Autodesk Inventor part; units mm, degrees
ref_plane "YZ Plane" through (0, 0, 0) normal (1, 0, 0) x (0, 1, 0)
ref_plane "XZ Plane" through (0, 0, 0) normal (0, 1, 0) x (-1, 0, 0)
ref_plane "XY Plane" through (0, 0, 0) normal (0, 0, 1) x (1, 0, 0)
sketch "Sketch1" plane through (0, 0, 0) normal (0, 1, 0) x (-1, 0, 0)
  line L0 (-9.1057, 3.648) -> (-9.1057, -9.552)
  line L1 (4.8943, -9.552) -> (4.8943, 8.308)
  line L2 (4.8943, 8.308) -> (-9.1057, 3.648)
  line L3 (-2.1057, 5.978) -> (-2.1057, 1.978)
  circle A0 centre (-2.1057, 0.378) radius 1.6
  line L4 (4.8943, -9.552) -> (4.8943, -12.052)
  line L5 (-9.1057, -9.552) -> (-9.1057, -12.052)
  line L6 (4.8943, -12.052) -> (-9.1057, -12.052)
  circle A1 centre (-2.1057, -12.052) radius 4
  line L7 (-2.1057, -1.222) -> (-2.1057, -8.052)
  line L8 (4.8943, 1.978) -> (-2.1057, 1.978)
  line L9 (-9.1057, 1.978) -> (-2.1057, 1.978)
  point P0 (0, 0)
  point P1 (1.8943, -12.052)
  point P2 (-6.1057, -12.052)
  dimension "d8" = 3.2
  dimension "d19" = 8
  dimension "d5" = 13.2
  dimension "d6" = 4
  dimension "d10" = 17.86
  dimension "d13" = 14
  dimension "d16" = 2.5
extrude "Extrusion2" add sketch "Sketch1" along normal blind 4 contours L2 L3 L9 L0 | L9 A0 L7 A1 L6 L5 L0 | L2 L1 L8 L3 | L8 L1 L4 L6 A1 L7 A0
sketch "Sketch2" plane through (0, 0, 0) normal (0, -1, 0) x (1, 0, 0)
  line L0 (9.1057, 3.648) -> (9.1057, -12.052)
  line L1 (9.1057, 2.0387) -> (-4.8943, 2.0387)
  line L2 (-4.8943, -12.052) -> (-4.8943, 8.308)
  line L3 (-4.8943, 2.0387) -> (-4.8943, 8.308)
  line L4 (-4.8943, 8.308) -> (9.1057, 3.648)
  line L5 (-4.8943, 8.308) -> (9.1057, 3.648)
  line L6 (9.1057, 3.648) -> (9.1057, 2.0387)
  point P0 (0, 0)
extrude "Extrusion3" add sketch "Sketch2" against normal blind 6
properties part number "plungerholdermod2"
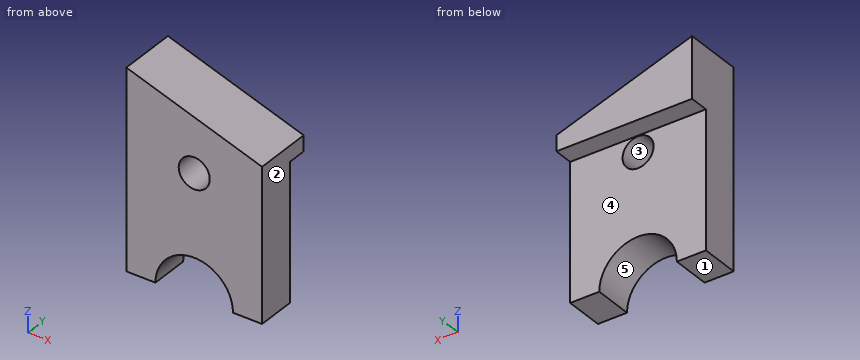
CAD build for the part. Positions are in the model's coordinates, mm. Face numbers are marked on the shaded views. A direction names the side the tool comes from. Round coordinates to 2 decimals unless told otherwise and drop trailing zeros. Order: outer loops, then holes, each group sorted by start corner. A loop starts at its lowest first (then second) coordinate and runs counter-clockwise, first axis right, second up. Notation, with made-up numbers: (5.5, 2) - (25.5, 2) arc R16 cw to (25.5, 16) - close; hole circle Ø6 at (-31, 83.5). An arc over 180 degrees is marked (long way). Return JSON: item names as keys, results as strings.
(1) Pull direction X, two halves, no side cores. Call the marked faces 1, 2 and 3: +X half, -X half, draft (parallel to the pull), parting line (faces both ways), or undercut.
Answer key:
{"face 1": "draft", "face 2": "+X half", "face 3": "undercut"}
(2) Tool access for the marked faces 4 and 5: list every direction of +Z, -Z, +X, -X, +Y, -Y with a clear straight run to the whole face (end or side of a thin tool).
Answer key:
{"face 4": "-Z, +X, -X, +Y", "face 5": "-Z, +Y, -Y"}
(3) Cut at C-C (z = -8.75). Give the cut face in (x, y).
Answer key:
{"outline": "(-4.89, 0) - (-0.15, 0) - (-0.15, 4) - (-4.89, 4) - close; (4.36, 0) - (9.11, 0) - (9.11, 4) - (4.36, 4) - close"}
(4) Cut at A-A (x = 3). Give the cut face in (y, z).
Answer key:
{"outline": "(0, -8.15) - (4, -8.15) - (4, -0.95) - (0, -0.95) - close; (0, 1.7) - (4, 1.7) - (4, 2.04) - (6, 2.04) - (6, 5.68) - (0, 5.68) - close"}
(5) Cut at D-D (x = 6.5). Give the cut face in (y, z), then the cut area to 3 significant figures.
Answer key:
{"outline": "(0, -12.05) - (4, -12.05) - (4, 2.04) - (6, 2.04) - (6, 4.52) - (0, 4.52) - close", "area": "71.2 mm^2"}
(6) Cut at B-B (y = 1.9). Give the cut face in (x, z).
Answer key:
{"outline": "(-4.89, -12.05) - (-1.89, -12.05) arc R4 cw to (6.11, -12.05) - (9.11, -12.05) - (9.11, 3.65) - (-4.89, 8.31) - close; hole circle Ø3.2 at (2.11, 0.38)"}
(7) Pin check, flat tips, straight feed: pin 1 Ø1 at (x, y) = (4.5, 3.5) entering from -Z; pin 2 Ø4 at (x, z) = (6.5, -3) entering from +Y; pin 3 Ø2.5 at (x, z) = (2.11, 0.38) entering from -Y; pin 4 Ø0.6 at (x, y) = (2.5, 4.5) entering from -Z. Stop position of each tip, or through.
Answer key:
{"pin 1": "stops at z = -9.29", "pin 2": "stops at y = 4", "pin 3": "passes through", "pin 4": "stops at z = 2.04"}
(8) Wall check: probe 1 along Y at (x, z) = (2, -1.5); probe 2 along X at (y, z) = (3.15, 0); probe 3 along Z at (x, y) = (8.5, 3.45). Give the ranges that are in metal, low to high. Write a range as from..to.
Answer key:
{"probe 1": "y = 0..4", "probe 2": "x = -4.89..0.55, 3.66..9.11", "probe 3": "z = -12.05..3.85"}
